Design review of the part shown in the three views and the two pictorial views. Dimensions are in mm from the part's minimum x, y and z. A direction names the side the tool comes from. Coordinates: 2 decimals unless noted, no trailing zeros. Loops run counter-clockwise (first coordinate to the right, second up) from the corner with the lowest first, then second, coordinate; pieces in that order, holes last. Notation, with made-up numbers: (8, 6.5) - (20, 6.5) arc R21 ccw to (20, 16.5) - close; hole circle Ø1 at (-18.5, 64). An arc over 180 degrees is marked (long way). One line per item, written item: value. Start each with the question number.
1. Take a section at B-B, the plane y = 8. State the section outline as (x, z) points, and give its area (3 significant figures).
2. Take a section at C-C, the plane z = 57.5. State the section outline as (x, y) points, and give its area (3 significant figures).
3. For the marked faces 1 and 2, list the 3-axis set-ups (+Z, -Z, +X, -X, +Y, -Y) from which the entire face can be reached by the end or side of a thin tool; tool diameter is ignored.
4. To check wall thickness, follow line 1 (Z direction, x = 13, y = 2.25); line 2 (X direction, y = 6.25, z = 54.5). State the ranges of each line that lie inside material, in increasing order. Write a range as from..to.
5. The part is to be moulded in two halves that separate along Z. For the marked faces 3, 4 and 5, say which applies: released by +Z, released by -Z, zero draft, split by the parting line, or undercut.
6. Take a section at A-A, the plane x = 10. State the section outline as (y, z) points.
7. Insertion check: pin 1 (4 mm diameter, centred on x = 27, z = 22, fed in from -Y). The pin has a flat end and moves straight along its axis. Give the tip position at first contact, or say it passes through.
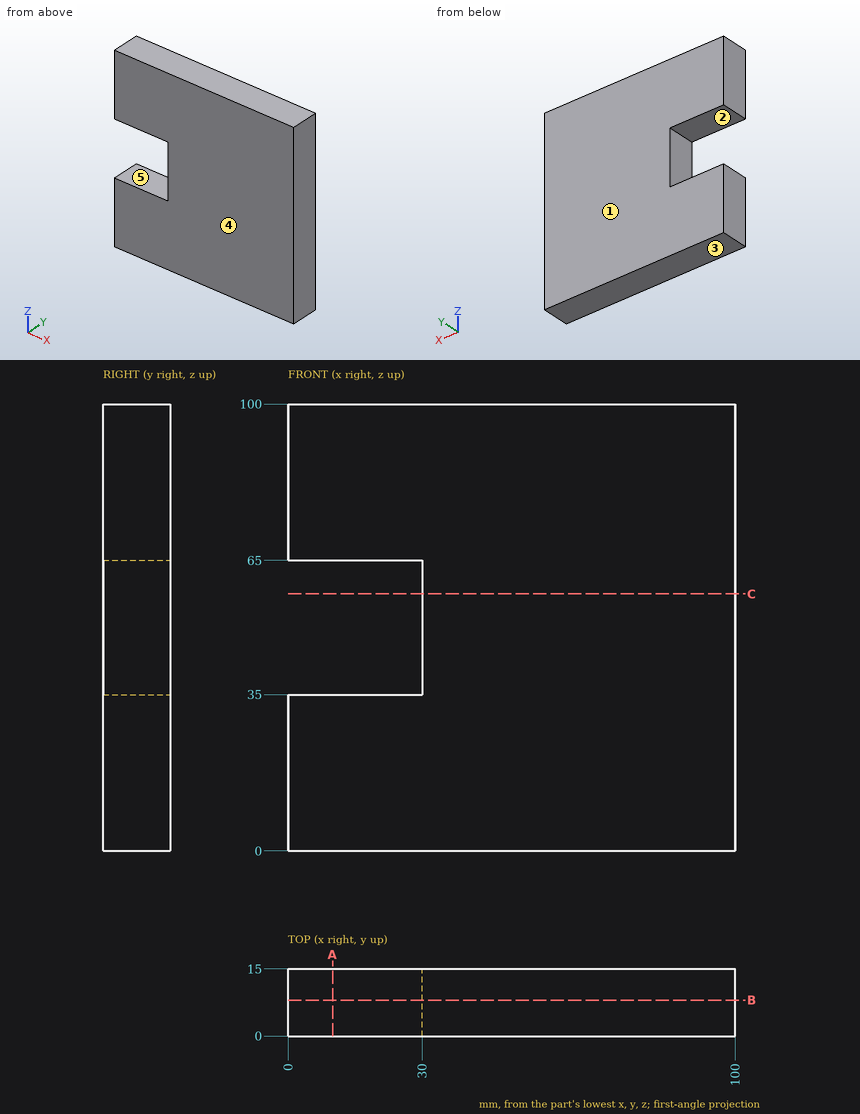
Solutions:
1. outline: (0, 0) - (100, 0) - (100, 100) - (0, 100) - (0, 65) - (30, 65) - (30, 35) - (0, 35) - close
1. area: 9,100 mm2
2. outline: (30, 0) - (100, 0) - (100, 15) - (30, 15) - close
2. area: 1,050 mm2
3. face 1: +Z, -Z, +X, -X, +Y
3. face 2: -X, +Y, -Y
4. line 1: 0..35, 65..100
4. line 2: 30..100
5. face 3: released by -Z
5. face 4: zero draft
5. face 5: undercut
6. outline: (0, 0) - (15, 0) - (15, 35) - (0, 35) - close; (0, 65) - (15, 65) - (15, 100) - (0, 100) - close
7. pin 1: y = 0
